from build123d import *

# Parameters (mm, degrees)
SKETCH_W     = 80
SKETCH_H     = 50
PAD_DEPTH    = 3
SKETCH001_W  = 72
SKETCH001_H  = 42
PAD001_DEPTH = 3
FILLET_R     = 6
SKETCH002_W  = 8
SKETCH002_H  = 8
PAD002_DEPTH = 8
FILLET001_R  = 3
SKETCH003_R  = 1.55
POCKET_DEPTH = 76.001


with BuildPart() as part:
    # Sketch → Pad (new body)
    with BuildSketch(Plane.XY):
        with Locations((-40, 25)):
            Rectangle(SKETCH_W, SKETCH_H)
    extrude(amount=PAD_DEPTH)

    # Sketch001 (on Face6 of Pad) → Pad001 (join)
    with BuildSketch(Plane.XY.offset(3)):
        with Locations((-40, 25)):
            Rectangle(SKETCH001_W, SKETCH001_H)
    extrude(amount=PAD001_DEPTH)

    # Fillet
    fillet_edges = [part.edges().sort_by_distance(p)[0] for p in [
        (-80, 0, 1.5),
        (-76, 4, 4.5),
        (-4, 4, 4.5),
        (0, 0, 1.5),
        (0, 50, 1.5),
        (-4, 46, 4.5),
        (-76, 46, 4.5),
        (-80, 50, 1.5),
    ]]
    fillet(fillet_edges, radius=FILLET_R)

    # Sketch002 (on Face19 of Fillet) → Pad002 (join)
    with BuildSketch(Plane.XY.offset(6)):
        with Locations((-72, 25)):
            Rectangle(SKETCH002_W, SKETCH002_H)
        with Locations((-8, 25)):
            Rectangle(SKETCH002_W, SKETCH002_H)
    extrude(amount=PAD002_DEPTH)

    # Fillet001
    fillet001_edges = [part.edges().sort_by_distance(p)[0] for p in [
        (-8, 21, 14),
        (-8, 29, 14),
        (-72, 21, 14),
        (-72, 29, 14),
    ]]
    fillet(fillet001_edges, radius=FILLET001_R)

    # Sketch003 (on Face29 of Fillet001) → Pocket (cut, through all)
    with BuildSketch(Plane.YZ.offset(-4)):
        with Locations((25, 11)):
            Circle(SKETCH003_R)
    extrude(amount=-POCKET_DEPTH, mode=Mode.SUBTRACT)


solid = part.part
Can you work these out from the model? Positions are in its coordinate system, mm. A direction names the side the tool comes from. Give positions to 0.01 mm unless a question says otherwise; leave off trailing zeros. Write each loop counter-clockwise with the first axis right and the second up, starting at its lowest first coordinate (ties: lowest second). Pieces come first, ordered by that corner, then holes. Notation, with made-up numbers: M 61,12.5 L 92,12.5 A11 cw 92,33.5 Z; hole C 86.25,34.25 d10. An arc over 180 degrees is marked long. Answer in a Markdown table with one row per item. Add a question column.
Item 1: Please list where these lines run through material, in increasing order: L1, parallel to X at y = 27, z = 9.5; L2, parallel to Z at x = -72.25, y = 25; L3, parallel to Y at x = -32.5, z = 5.
Item 2: Imagine slicing it at A-A, the plane z = 8.5. Write out the boundary of the cut face in (x, y), plus the area to 3 significant figures.
Item 3: On a 3-axis mill with a long thin cutter (end or side, diameter ignored), from which of +Z, -Z, +X, -X, +Y, -Y can I reach the whole of each face in a straight line? I mean faces 4 (the flat face through (-4, 25, 6)), 5 (the cylindrical face through (-74.196, 5.711, 4.521)), 6 (the cylindrical face through (-74.196, 44.289, 4.521)). Say none if no direction works.
Item 4: We'd pull the mould along X, two halves only. Please class faces 1 (the flat face through (-80, 25, 1)), 2 (the flat face through (-40, 46, 4)), 3 (the flat face through (-68, 25, 9)): released by +X, released by -X, zero draft, split by the parting line, or undercut.
Item 5: Imagine slicing it at B-B, the plane y = 25. Write out the boundary of the cut face in (x, z).
Item 6: For pin 1 Ø4 at (y, z) = (25, 11) entering from -X; pin 2 Ø1 at (x, z) = (-48.5, 4.5) entering from +Y; pin 3 Ø1.5 at (x, z) = (-8, 7.5) entering from -Y, each with a flat end and sliding along its axis, tell me the tip position at first contact or that it passes through.
Item 7: Imagine slicing it at C-C, the plane x = -47.5. Write out the boundary of the cut face in (y, z), plus the area to 3 significant figures.
Item 8: Imagine slicing it at D-D, the plane y = 15. Write out the boundary of the cut face in (x, z), plus the area to 3 significant figures.
Evaluation:
| question | item | result |
|---|---|---|
| 1 | L1 | x = -76 to -68, -12 to -4 |
| 1 | L2 | z = 0 to 9.45, 12.55 to 14 |
| 1 | L3 | y = 4 to 46 |
| 2 | outline | M -76,21 L -68,21 L -68,29 L -76,29 Z; M -12,21 L -4,21 L -4,29 L -12,29 Z |
| 2 | area | 128 mm² |
| 3 | face 4 | +Z, +X, +Y, -Y |
| 3 | face 5 | +Z, -X, -Y |
| 3 | face 6 | +Z, -X, +Y |
| 4 | face 1 | released by -X |
| 4 | face 2 | zero draft |
| 4 | face 3 | undercut |
| 5 | outline | M -80,0 L 0,0 L 0,3 L -4,3 L -4,9.45 L -12,9.45 L -12,6 L -68,6 L -68,9.45 L -76,9.45 L -76,3 L -80,3 Z; M -76,12.55 L -68,12.55 L -68,14 L -76,14 Z; M -12,12.55 L -4,12.55 L -4,14 L -12,14 Z |
| 6 | pin 1 | stops at x = -76 |
| 6 | pin 2 | stops at y = 46 |
| 6 | pin 3 | stops at y = 21 |
| 7 | outline | M 0,0 L 50,0 L 50,3 L 46,3 L 46,6 L 4,6 L 4,3 L 0,3 Z |
| 7 | area | 276 mm² |
| 8 | outline | M -80,0 L 0,0 L 0,3 L -4,3 L -4,6 L -76,6 L -76,3 L -80,3 Z |
| 8 | area | 456 mm² |
